Geometry: final body of the model. Coordinates: model frame, mm. A direction names the side the tool comes from. Give positions to 0.01 mm unless a question says otherwise; leave off trailing zeros. Write each loop counter-clockwise with the first axis right and the second up, starting at its lowest first coordinate (ties: lowest second). Pieces come first, ordered by that corner, then holes. Notation, with made-up numbers: (28.25, -29) -> (62.25, -29) arc R21 ccw to (62.25, -6) -> close; hole circle Ø9 at (-20, 83.5). An arc over 180 degrees is marked (long way). Answer in a Markdown table with one row per item. Add a question column.
from build123d import *

# Parameters (mm, degrees)
SKETCH_1_W          = 188
SKETCH_1_H          = 108
EXTRUDE_1_DEPTH     = 8
SKETCH_2_R          = 2.95
SKETCH_2_W          = 128
SKETCH_2_H          = 96
CUT_EXTRUDE_1_DEPTH = 9
FILLET_1_R          = 3


with BuildPart() as part:
    # Эскиз1 → Бобышка-Вытянуть1 (new body)
    with BuildSketch(Plane(origin=(0, 0, 0), x_dir=(1, 0, 0), z_dir=(0, 1, 0))):
        Rectangle(SKETCH_1_W, SKETCH_1_H)
    extrude(amount=EXTRUDE_1_DEPTH)

    # Эскиз2 → Вырез-Вытянуть1 (cut, through all)
    with BuildSketch(Plane(origin=(0, 8, 0), x_dir=(1, 0, 0), z_dir=(0, 1, 0))):
        with Locations((-73, 44)):
            Circle(SKETCH_2_R)
        with Locations((73, 44)):
            Circle(SKETCH_2_R)
        with Locations((-73, -44)):
            Circle(SKETCH_2_R)
        with Locations((73, -44)):
            Circle(SKETCH_2_R)
        with Locations((1.5, 0)):
            Rectangle(SKETCH_2_W, SKETCH_2_H)
    extrude(amount=-CUT_EXTRUDE_1_DEPTH, mode=Mode.SUBTRACT)

    # Скругление1
    fillet_1_edges = [part.edges().sort_by_distance(p)[0] for p in [
        (65.5, 4, -48),
        (65.5, 4, 48),
        (-62.5, 4, 48),
        (-62.5, 4, -48),
    ]]
    fillet(fillet_1_edges, radius=FILLET_1_R)


solid = part.part
Q1. Section A-A on z = 14.5. Return loops of the section in (x, y), and give its area (3 significant figures).
Q2. Section D-D on x = -73. Return loops of the section in (y, z).
Q3. Section C-C on y = 5. Return loops of the section in (x, z), and give its area (3 significant figures).
Q4. Section B-B on x = -6.5. Return loops of the section in (y, z), and give its area (3 significant figures).
Q5. Line query: probe 1 along X at (y, z) = (4.5, 44); probe 2 along Z at (x, y) = (-73, 2); probe 3 along X at (y, z) = (6.75, -39). Output: solid intervals per line, ascending. Write a range as from..to.
Q6. Pull-direction query (Z, two-part tool) for faces 1 (the flat face through (-1, 4, 54)), 2 (the flat face through (94, 4, 1)), 3 (the flat face through (-62.5, 4, 1)); classes: +Z half, -Z half, draft (parallel to the pull), parting line (faces both ways), or undercut.
Q7. Access query for faces 4 (the flat face through (1, 4, 48)), 5 (the flat face through (-22, 8, -49)). Directions: +Z, -Z, +X, -X, +Y, -Y. A direction counts if a zero-diameter tool reaches every point of the face in a straight line with its end or side. Return the directions, or none.
Q8. Contact query for flat-ended pins moving along their axis: pin 1 Ø12 at (x, z) = (48.5, -43) entering from -Y; pin 2 Ø3.5 at (x, z) = (-73, 44) entering from -Y. Output: stop coordinate, or through.
Checks:
| question | item | result |
|---|---|---|
| 1 | outline | (-94, 0) -> (-62.5, 0) -> (-62.5, 8) -> (-94, 8) -> close; (65.5, 0) -> (94, 0) -> (94, 8) -> (65.5, 8) -> close |
| 1 | area | 480 mm^2 |
| 2 | outline | (0, -54) -> (8, -54) -> (8, -46.95) -> (0, -46.95) -> close; (0, -41.05) -> (8, -41.05) -> (8, 41.05) -> (0, 41.05) -> close; (0, 46.95) -> (8, 46.95) -> (8, 54) -> (0, 54) -> close |
| 3 | outline | (-94, -54) -> (94, -54) -> (94, 54) -> (-94, 54) -> close; hole circle Ø5.9 at (-73, -44); hole circle Ø5.9 at (-73, 44); hole (-62.5, -45) arc R3 ccw to (-59.5, -48) -> (62.5, -48) arc R3 ccw to (65.5, -45) -> (65.5, 45) arc R3 ccw to (62.5, 48) -> (-59.5, 48) arc R3 ccw to (-62.5, 45) -> close; hole circle Ø5.9 at (73, -44); hole circle Ø5.9 at (73, 44) |
| 3 | area | 7,910 mm^2 |
| 4 | outline | (0, -54) -> (8, -54) -> (8, -48) -> (0, -48) -> close; (0, 48) -> (8, 48) -> (8, 54) -> (0, 54) -> close |
| 4 | area | 96.0 mm^2 |
| 5 | probe 1 | -94..-75.95, -70.05..-62.5, 65.5..70.05, 75.95..94 |
| 5 | probe 2 | -54..-46.95, -41.05..41.05, 46.95..54 |
| 5 | probe 3 | -94..-62.5, 65.5..94 |
| 6 | face 1 | +Z half |
| 6 | face 2 | draft |
| 6 | face 3 | undercut |
| 7 | face 4 | +Y, -Y |
| 7 | face 5 | +Z, -Z, +X, -X, +Y |
| 8 | pin 1 | y = 0 |
| 8 | pin 2 | through |
